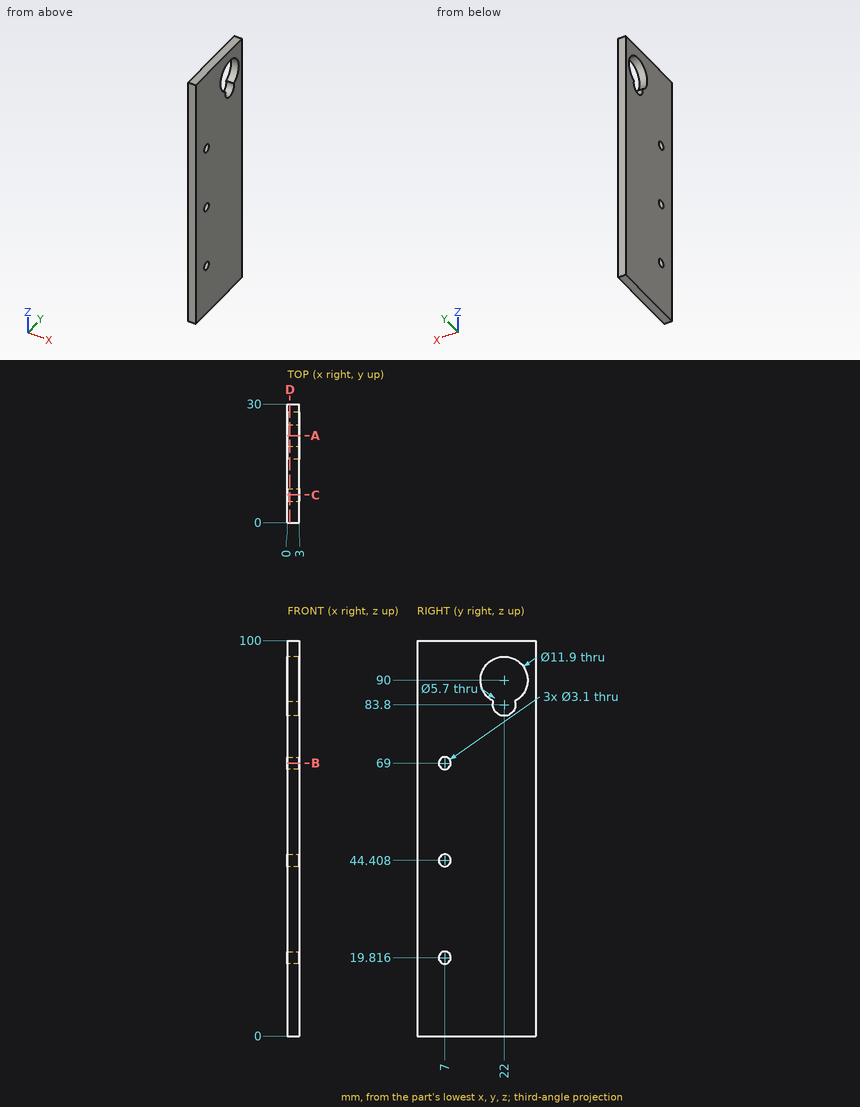
Check sheet for the drawn part. Datum: minimum x, y, z corner. Units: mm. Round coordinates to 2 decimals unless told otherwise and drop trailing zeros. Order: outer loops, then holes, each group sorted by start corner. A loop starts at its lowest first (then second) coordinate and runs counter-clockwise, first axis right, second up. Notation, with made-up numbers: (70.25, 13) -> (120.25, 13) arc R6 ccw to (120.25, 23) -> close; hole circle Ø8 at (79, 75). An arc over 180 degrees is marked (long way). Put each result on its own line as item: value. Start each with the question number.
(1) Section check C-C (y = 7). Enter the section's corners in (x, z).
(2) Section check B-B (z = 69). Enter the section's corners in (x, y), then the cut area to 3 significant figures.
(3) Depth check by flat-ended pin: pin 1 Ø4 at (y, z) = (25, 14.5) entering from -X. Enter the tip coordinate at first touch or a pass-through.
(4) Material ranges on line 1 along Z through (x, y) = (2.75, 22); line 2 along Z through (x, y) = (0.15, 6) (1 decimal); line 3 along Y through (x, z) = (1.4, 69), recorded low to high.
(5) Section check A-A (y = 22). Enter the section's corners in (x, z), then the cut area to 3 significant figures.
(6) Section check D-D (x = 0.65). Enter the section's corners in (y, z), then the cut area to 3 significant figures.
Completed:
1. outline: (0, 0) -> (3, 0) -> (3, 18.27) -> (0, 18.27) -> close; (0, 21.37) -> (3, 21.37) -> (3, 42.86) -> (0, 42.86) -> close; (0, 45.96) -> (3, 45.96) -> (3, 67.45) -> (0, 67.45) -> close; (0, 70.55) -> (3, 70.55) -> (3, 100) -> (0, 100) -> close
2. outline: (0, 0) -> (3, 0) -> (3, 5.45) -> (0, 5.45) -> close; (0, 8.55) -> (3, 8.55) -> (3, 30) -> (0, 30) -> close
2. area: 80.7 mm2
3. pin 1: stops at x = 0
4. line 1: z = 0 to 80.95, 95.95 to 100
4. line 2: z = 0 to 18.6, 21 to 43.2, 45.6 to 67.8, 70.2 to 100
4. line 3: y = 0 to 5.45, 8.55 to 30
5. outline: (0, 0) -> (3, 0) -> (3, 80.95) -> (0, 80.95) -> close; (0, 95.95) -> (3, 95.95) -> (3, 100) -> (0, 100) -> close
5. area: 255 mm2
6. outline: (0, 0) -> (30, 0) -> (30, 100) -> (0, 100) -> close; hole circle Ø3.1 at (7, 19.82); hole circle Ø3.1 at (7, 44.41); hole circle Ø3.1 at (7, 69); hole (19.3, 84.7) arc R2.85 ccw (long way) to (24.7, 84.7) arc R5.95 ccw (long way) to start
6. area: 2,850 mm2
